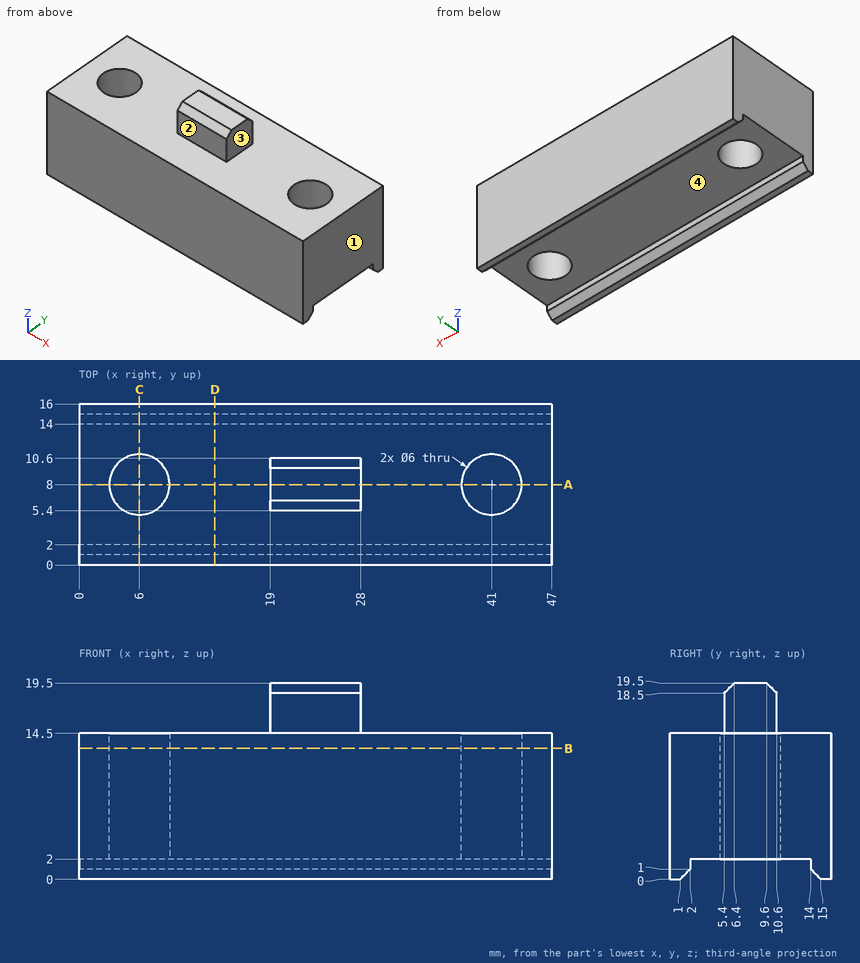
Source: three-view drawing plus pictorial views. Frame: mm from the lowest corner of the part. A direction names the side the tool comes from. Round coordinates to 2 decimals unless told otherwise and drop trailing zeros. Write each loop counter-clockwise with the first axis right and the second up, starting at its lowest first coordinate (ties: lowest second). Pieces come first, ordered by that corner, then holes. Notation, with made-up numbers: (-32.5, 53) -> (11.5, 53) arc R21 ccw to (11.5, 83) -> close; hole circle Ø7 at (42.5, -21.75). An arc over 180 degrees is marked (long way). Return JSON: item names as keys, results as strings.
Q1. First-contact query: pin 1 Ø1 at (x, y) = (31.5, 10) entering from +Z; pin 2 Ø2 at (x, z) = (24, 16) entering from +Y; pin 3 Ø2.5 at (y, z) = (9, 17) entering from +X; pin 4 Ø3.5 at (x, y) = (41, 8) entering from -Z. Flat tips, straight axial feed; report the tip coordinate or a pass-through.
From the geometry:
{"pin 1": "z = 14.5", "pin 2": "y = 10.6", "pin 3": "x = 28", "pin 4": "through"}
Q2. Ray query, line 1 (Y direction, x = 6, z = 11.75); line 2 (Y direction, x = 35, z = 1.5); line 3 (Z direction, x = 34.5, y = 13). Return the intervals inside material, ascending.
From the geometry:
{"line 1": "0 to 5, 11 to 16", "line 2": "0 to 2, 14 to 16", "line 3": "2 to 14.5"}
Q3. Section D-D on x = 13.5. Return the cut outline in (y, z).
From the geometry:
{"outline": "(0, 0) -> (1, 0) -> (2, 1) -> (2, 2) -> (14, 2) -> (14, 1) -> (15, 0) -> (16, 0) -> (16, 14.5) -> (0, 14.5) -> close"}
Q4. Section A-A on y = 8. Return the cut outline in (x, z), and give its area (4 significant figures).
From the geometry:
{"outline": "(0, 2) -> (3, 2) -> (3, 14.5) -> (0, 14.5) -> close; (9, 2) -> (38, 2) -> (38, 14.5) -> (28, 14.5) -> (28, 19.5) -> (19, 19.5) -> (19, 14.5) -> (9, 14.5) -> close; (44, 2) -> (47, 2) -> (47, 14.5) -> (44, 14.5) -> close", "area": "482.5 mm2"}
Q5. Section B-B on z = 13. Return the cut outline in (x, y).
From the geometry:
{"outline": "(0, 0) -> (47, 0) -> (47, 16) -> (0, 16) -> close; hole circle Ø6 at (6, 8); hole circle Ø6 at (41, 8)"}
Q6. Set-up query: the marked faces 1, 2, 3 and 4. Return all of +Z, -Z, +X, -X, +Y, -Y with unobstructed straight access to the full face (end or side cutting, diameter ignored); none if empty.
From the geometry:
{"face 1": "+Z, -Z, +X, +Y, -Y", "face 2": "+Z, +X, -X, -Y", "face 3": "+Z, +X, +Y, -Y", "face 4": "-Z, +X, -X"}
Q7. Section C-C on x = 6. Return the cut outline in (y, z).
From the geometry:
{"outline": "(0, 0) -> (1, 0) -> (2, 1) -> (2, 2) -> (5, 2) -> (5, 14.5) -> (0, 14.5) -> close; (11, 2) -> (14, 2) -> (14, 1) -> (15, 0) -> (16, 0) -> (16, 14.5) -> (11, 14.5) -> close"}
